```python
from build123d import *

# Parameters (mm, degrees)
SKETCH2_W            = 52.8
SKETCH2_H            = 12
BASE_FLANGE1_DEPTH   = 0.05
EDGE_FLANGE1_START   = -6
EDGE_FLANGE1_DEPTH   = 12
EDGE_FLANGE1_2_DEPTH = 12
CUT_EXTRUDE2_DEPTH   = 0.05
SKETCH10_R           = 1.6
CUT_EXTRUDE1_DEPTH   = 31.402652498
FILLET1_R            = 0.5


# Read off the part's stored shape, not the designer's step: Edge-Flange1
# Sheet-metal steps are written as plain solids
with BuildPart() as part:
    # Sketch2 → Base-Flange1 (new body)
    with BuildSketch(Plane(origin=(0, 0, 0), x_dir=(1, 0, 0), z_dir=(0, 1, 0))):
        Rectangle(SKETCH2_W, SKETCH2_H)
    extrude(amount=-BASE_FLANGE1_DEPTH)

    # Edge-Flange1 outline → Edge-Flange1 (cut)
    with BuildSketch(Plane.XY.offset(EDGE_FLANGE1_START)):
        with BuildLine():
            ThreePointArc((25.929678854, 0), (26.046939248, -0.012645368), (26.158807639, -0.05))
            Line((26.158807639, -0.05), (26.4, -0.05))
            Line((26.4, -0.05), (26.4, 0))
            Line((26.4, 0), (25.929678854, 0))
        make_face()
    extrude(amount=EDGE_FLANGE1_DEPTH, mode=Mode.SUBTRACT)

    # Edge-Flange1 2 outline → Edge-Flange1 2 (add)
    with BuildSketch(Plane.XY.offset(EDGE_FLANGE1_START)):
        with BuildLine():
            Line((28.127665428, -9.84807753), (26.471323118, -0.454493502))
            ThreePointArc((26.471323118, -0.454493502), (26.364910426, -0.213735999), (26.158807639, -0.05))
            Line((26.158807639, -0.05), (25.929678854, -0.05))
            ThreePointArc((25.929678854, -0.05), (26.251072659, -0.166977778), (26.42208273, -0.463175911))
            Line((26.42208273, -0.463175911), (28.07842504, -9.856759939))
            Line((28.07842504, -9.856759939), (28.127665428, -9.84807753))
        make_face()
    extrude(amount=EDGE_FLANGE1_2_DEPTH)

    # Sketch11 → Cut-Extrude2 (cut)
    with BuildSketch(Plane(origin=(25.595392091, 4.513158207, 0), x_dir=(0, 0, -1), z_dir=(0.9848077530122074, 0.17364817766693416, 0))):
        Polygon((29.405769939, -61.330580197), (0, -14.582780947), (-6, -5.044285745), (-6, -14.582780947), (-6, -69.810093397), (19.725851686, -177.227060012), (55.131621625, -168.747546812), align=None)
    cut_extrude2 = extrude(amount=-CUT_EXTRUDE2_DEPTH, mode=Mode.SUBTRACT)

    # Mirror1: Cut-Extrude2 across plane
    add(cut_extrude2.mirror(Plane.XY), mode=Mode.SUBTRACT)

    # Sketch10 → Cut-Extrude1 (cut, through all)
    with BuildSketch(Plane(origin=(0, 0, 0), x_dir=(1, 0, 0), z_dir=(0, 1, 0))):
        with Locations(Location((-22.4, 3, 0), (0, 0, 270))):
            Circle(SKETCH10_R)
        with Locations(Location((-22.4, -3, 0), (0, 0, 270))):
            Circle(SKETCH10_R)
    extrude(amount=-CUT_EXTRUDE1_DEPTH, mode=Mode.SUBTRACT)

    # Fillet1
    fillet1_edges = [part.edges().sort_by_distance(p)[0] for p in [
        (-26.4, -0.025, 6),
        (-26.4, -0.025, -6),
    ]]
    fillet(fillet1_edges, radius=FILLET1_R)


solid = part.part
```
Work out the finished part from the listing and answer in its coordinate system (mm). Round coordinates to 2 decimals unless told otherwise and drop trailing zeros. Loops run counter-clockwise (first coordinate to the right, second up) from the corner with the lowest first, then second, coordinate; pieces in that order, holes last. Notation, with made-up numbers: (-20.75, 41.5) -> (17.25, 41.5) arc R21 cw to (17.25, 53.5) -> close; hole circle Ø5 at (31.5, 70.25). An arc over 180 degrees is marked (long way). Write each question's results on one line, items separated by ' | '. Start each with the question number.
1. Section D-D (z = 2) is taken. Determine the outline of the cut face in (x, y).
2. Given pin 1 Ø1 at (y, z) = (-7.5, 3) entering from +X; pin 2 Ø4 at (y, z) = (-7.5, -0.5) entering from -X; pin 3 Ø5 at (y, z) = (-8.5, 1) entering from +X, each flat-ended and moving along its own axis, determine where each tip first touches the part or whether it passes through.
3. Section B-B (z = -3.5) is taken. Determine the outline of the cut face in (x, y).
4. Section A-A (x = -22.4) is taken. Determine the outline of the cut face in (y, z).
5. Section C-C (x = -13) is taken. Determine the outline of the cut face in (y, z), plus the area to 3 significant figures.
Evaluation:
1) outline: (-26.4, -0.05) -> (-23.65, -0.05) -> (-23.65, 0) -> (-26.4, 0) -> close; (-21.15, -0.05) -> (25.93, -0.05) arc R0.5 cw to (26.42, -0.46) -> (27.53, -6.73) -> (27.58, -6.72) -> (26.47, -0.45) arc R0.55 ccw to (25.93, 0) -> (-21.15, 0) -> close
2) pin 1: passes through | pin 2: stops at x = 27.31 | pin 3: stops at x = 28.13
3) outline: (-26.4, -0.05) -> (-23.92, -0.05) -> (-23.92, 0) -> (-26.4, 0) -> close; (-20.88, -0.05) -> (25.93, -0.05) arc R0.5 cw to (26.42, -0.46) -> (27.11, -4.38) -> (27.16, -4.37) -> (26.47, -0.45) arc R0.55 ccw to (25.93, 0) -> (-20.88, 0) -> close
4) outline: (-0.05, -6) -> (0, -6) -> (0, -4.6) -> (-0.05, -4.6) -> close; (-0.05, -1.4) -> (0, -1.4) -> (0, 1.4) -> (-0.05, 1.4) -> close; (-0.05, 4.6) -> (0, 4.6) -> (0, 6) -> (-0.05, 6) -> close
5) outline: (-0.05, -6) -> (0, -6) -> (0, 6) -> (-0.05, 6) -> close | area: 0.600 mm2
